For this review, take the finished solid that the model builds, in its own axes (mm). Face numbers are marked on the shaded views. A direction names the side the tool comes from. Give positions to 0.01 mm unless a question says otherwise; leave off trailing zeros. Loops run counter-clockwise (first coordinate to the right, second up) from the corner with the lowest first, then second, coordinate; pieces in that order, holes last. Notation, with made-up numbers: (33, 70.25) -> (81, 70.25) arc R17 ccw to (81, 103.25) -> close; hole circle Ø5 at (22.25, 30). An arc over 180 degrees is marked (long way). Answer as CSV lines item,"result". Start each with the question number.
Item 1: For L1, parallel to Z at x = 0, y = 20.5; L2, parallel to X at y = 9, z = 50; L3, parallel to Z at x = 0, y = 7, list the stretches that pass through material, from the lowest coordinate up. Write a range as from..to.
Item 2: Add section C-C on x = -6. State the section outline as (y, z) points.
Item 3: Clearance check with flat-ended pins moving along their axes: P1, Ø8, axis at y = 4, z = -34.5, coming from the -X side; P2, Ø6, axis at x = 0, z = 100, coming from the +Y side; P3, Ø2, axis at x = 19, z = 67, coming from the -Y side; P4, Ø11, axis at x = 86.6, z = -50, coming from the +Y side. State where each tip first meets the part, or that it passes through.
Item 4: Add section B-B on z = 0. State the section outline as (x, y) points, plus the area to 3 significant figures.
Item 5: The part is to be moulded in two halves that separate along X. For the marked faces 1, 2 and 3, say which applies: +X half, -X half, draft (parallel to the pull), parting line (faces both ways), or undercut.
Item 6: Machinability: for the marked faces 4 and 5, which of the approach directions +Z, -Z, +X, -X, +Y, -Y give a long, thin tool a straight path to every point of the face, cutting with its end or side? Answer none if there is none.
Item 7: Add section A-A on y = 19.5. State the section outline as (x, z) points, plus the area to 3 significant figures.
Item 8: Add section D-D on z = 50. State the section outline as (x, y) points.
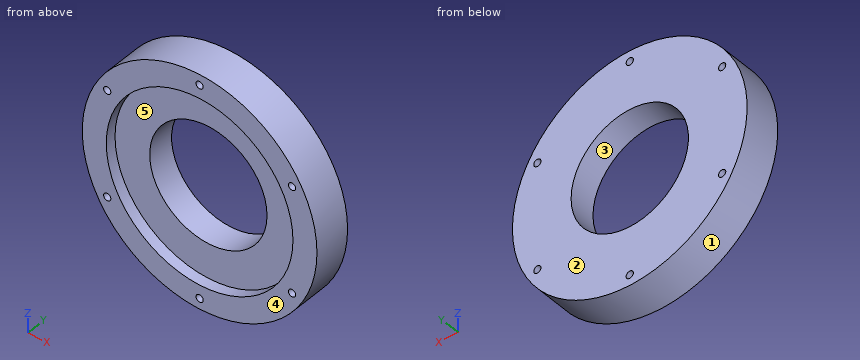
```python
from build123d import *

# Parameters (mm, degrees)
SKETCH1_R           = 110
SKETCH1_R_2         = 55
SKETCH1_R_3         = 3.4
BOSS_EXTRUDE1_DEPTH = 35
SKETCH2_R           = 87.5
CUT_EXTRUDE1_DEPTH  = 10


with BuildPart() as part:
    # Sketch1 → Boss-Extrude1 (new body)
    with BuildSketch(Plane(origin=(0, 0, 0), x_dir=(1, 0, 0), z_dir=(0, 1, 0))):
        Circle(SKETCH1_R)
        Circle(SKETCH1_R_2, mode=Mode.SUBTRACT)
        with Locations((0, 100)):
            Circle(SKETCH1_R_3, mode=Mode.SUBTRACT)
        with Locations((86.602540378, 50)):
            Circle(SKETCH1_R_3, mode=Mode.SUBTRACT)
        with Locations((86.602540378, -50)):
            Circle(SKETCH1_R_3, mode=Mode.SUBTRACT)
        with Locations((0, -100)):
            Circle(SKETCH1_R_3, mode=Mode.SUBTRACT)
        with Locations((-86.602540378, -50)):
            Circle(SKETCH1_R_3, mode=Mode.SUBTRACT)
        with Locations((-86.602540378, 50)):
            Circle(SKETCH1_R_3, mode=Mode.SUBTRACT)
    extrude(amount=BOSS_EXTRUDE1_DEPTH)

    # Sketch2 → Cut-Extrude1 (cut)
    with BuildSketch(Plane.XZ):
        Circle(SKETCH2_R)
    extrude(amount=-CUT_EXTRUDE1_DEPTH, mode=Mode.SUBTRACT)


solid = part.part
```
Computed values:
1,L1,"-110..-103.4, -96.6..-55, 55..96.6, 103.4..110"
1,L2,"-97.98..-90, -83.2..-71.81, 71.81..83.2, 90..97.98"
1,L3,"-110..-103.4, -96.6..-87.5, 87.5..96.6, 103.4..110"
2,outline,"(0, -109.84) -> (35, -109.84) -> (35, -54.67) -> (10, -54.67) -> (10, -87.29) -> (0, -87.29) -> close; (0, 87.29) -> (10, 87.29) -> (10, 54.67) -> (35, 54.67) -> (35, 109.84) -> (0, 109.84) -> close"
3,P1,"x = -105.69"
3,P2,"through"
3,P3,"y = 10"
3,P4,"y = 35"
4,outline,"(-110, 0) -> (-87.5, 0) -> (-87.5, 10) -> (-55, 10) -> (-55, 35) -> (-110, 35) -> close; (55, 10) -> (87.5, 10) -> (87.5, 0) -> (110, 0) -> (110, 35) -> (55, 35) -> close"
4,area,"3,200 mm²"
5,face 1,"parting line"
5,face 2,"draft"
5,face 3,"undercut"
6,face 4,"+Z, -Z, +X, -X, -Y"
6,face 5,"-Y"
7,outline,"circle Ø220 at (0, 0); hole circle Ø6.8 at (-86.6, -50); hole circle Ø6.8 at (-86.6, 50); hole circle Ø110 at (0, 0); hole circle Ø6.8 at (0, -100); hole circle Ø6.8 at (0, 100); hole circle Ø6.8 at (86.6, -50); hole circle Ø6.8 at (86.6, 50)"
7,area,"28,300 mm²"
8,outline,"(-97.98, 0) -> (-90, 0) -> (-90, 35) -> (-97.98, 35) -> close; (-83.2, 0) -> (-71.81, 0) -> (-71.81, 10) -> (-22.91, 10) -> (-22.91, 35) -> (-83.2, 35) -> close; (22.91, 10) -> (71.81, 10) -> (71.81, 0) -> (83.2, 0) -> (83.2, 35) -> (22.91, 35) -> close; (90, 0) -> (97.98, 0) -> (97.98, 35) -> (90, 35) -> close"
